Source: three-view drawing plus pictorial views. Frame: mm from the lowest corner of the part. A direction names the side the tool comes from. Give positions to 0.01 mm unless a question says otherwise; leave off trailing zeros. Loops run counter-clockwise (first coordinate to the right, second up) from the corner with the lowest first, then second, coordinate; pieces in that order, holes last. Notation, with made-up numbers: (-25, 13.5) - (-15, 13.5) arc R27 cw to (-15, 36.5) - close; hole circle Ø2 at (45, 57.25). An arc over 180 degrees is marked (long way). Answer in a Markdown table with one row per item.
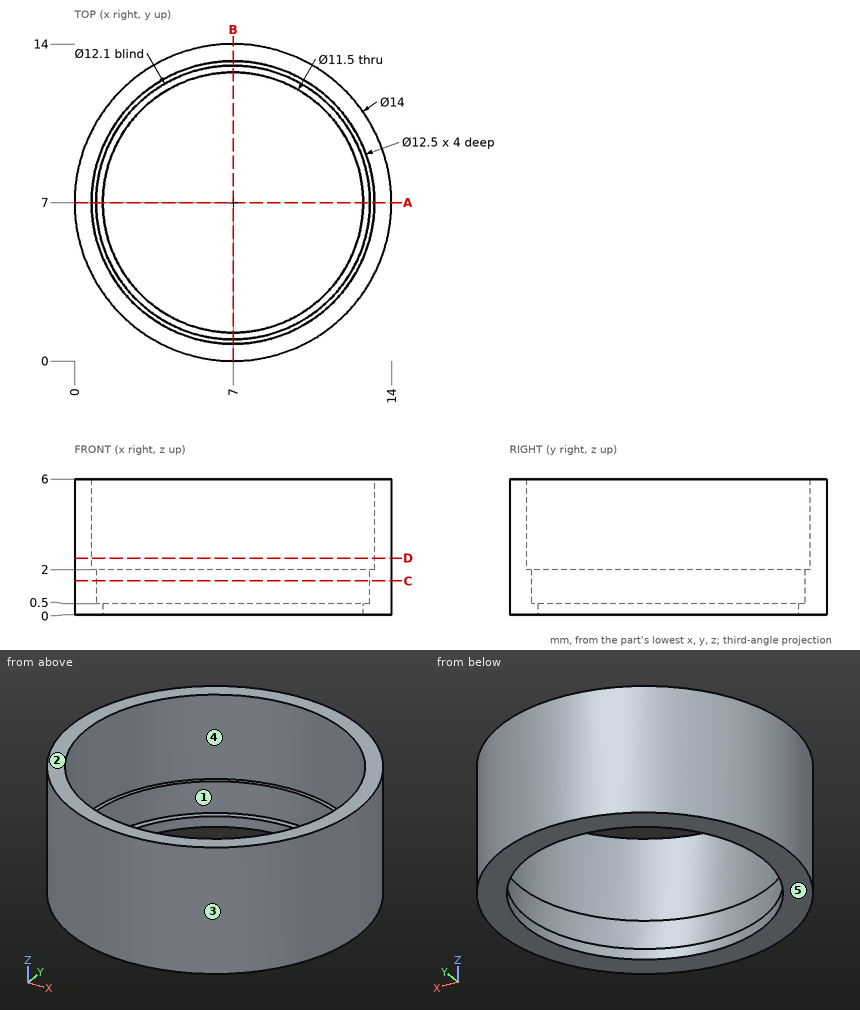
Q1. Reachability of the marked faces 4 and 5 from +Z, -Z, +X, -X, +Y, -Y: full face, straight path, thin tool, end or side. Return the list, or none.
Check values:
| item | result |
|---|---|
| face 4 | +Z |
| face 5 | -Z, +X, -X, +Y, -Y |
Q2. Cut plane A-A (y = 7). Output: boundary loops of the cut face in (x, z), and give its area (3 significant figures).
Check values:
| item | result |
|---|---|
| outline | (0, 0) - (1.25, 0) - (1.25, 0.5) - (0.95, 0.5) - (0.95, 2) - (0.75, 2) - (0.75, 6) - (0, 6) - close; (12.75, 0) - (14, 0) - (14, 6) - (13.25, 6) - (13.25, 2) - (13.05, 2) - (13.05, 0.5) - (12.75, 0.5) - close |
| area | 10.1 mm² |
Q3. First-contact query: pin 1 (3 mm diameter, centred on x = 12.5, z = 2.5, fed in from +Y); pin 2 (6 mm diameter, centred on x = 8, y = 6.5, fed in from +Z); pin 3 (2 mm diameter, centred on x = 3, z = 2.5, fed in from -Y). Flat tips, straight axial feed; report the tip coordinate or a pass-through.
Check values:
| item | result |
|---|---|
| pin 1 | y = 12.74 |
| pin 2 | through |
| pin 3 | y = 0.68 |
Q4. Material intervals for line 1 along Y through (x, z) = (7, 0.95); line 2 along Y through (x, z) = (7, 3.25); line 3 along Z through (x, y) = (12.75, 6.25), sorted ascending.
Check values:
| item | result |
|---|---|
| line 1 | 0 to 0.95, 13.05 to 14 |
| line 2 | 0 to 0.75, 13.25 to 14 |
| line 3 | 0 to 0.5 |
Q5. Cut plane D-D (z = 2.5). Output: boundary loops of the cut face in (x, y).
Check values:
| item | result |
|---|---|
| outline | circle Ø14 at (7, 7); hole circle Ø12.5 at (7, 7) |
Q6. Cut plane C-C (z = 1.5). Output: boundary loops of the cut face in (x, y), and give its area (3 significant figures).
Check values:
| item | result |
|---|---|
| outline | circle Ø14 at (7, 7); hole circle Ø12.1 at (7, 7) |
| area | 38.9 mm² |
Q7. Draft query along X for the marked faces 1, 2 and 3. Return one class per face: pulls with the +X half, pulls with the -X half, needs draft (parallel to the pull), parting line crosses it, or undercut.
Check values:
| item | result |
|---|---|
| face 1 | undercut |
| face 2 | needs draft |
| face 3 | parting line crosses it |
